```python
from build123d import *

# Parameters (mm, degrees)
F0_R     = 1.75
F0_R_2   = 2.75
F0_R_3   = 19.25
F1_DEPTH = 8
F2_R     = 3
F3_DEPTH = 3.5


with BuildPart() as f1:
    # F0 (on Right) → F1 (new body)
    with BuildSketch(Plane.YZ):
        with BuildLine():
            ThreePointArc((4.242641, 45.254834), (0, 47.012193), (-4.242641, 45.254834))
            Line((-4.242641, 45.254834), (-45.254834, 4.242641))
            ThreePointArc((-45.254834, 4.242641), (-47.012193, 0), (-45.254834, -4.242641))
            Line((-45.254834, -4.242641), (-4.242641, -45.254834))
            ThreePointArc((-4.242641, -45.254834), (0, -47.012193), (4.242641, -45.254834))
            Line((4.242641, -45.254834), (45.254834, -4.242641))
            ThreePointArc((45.254834, -4.242641), (47.012193, 0), (45.254834, 4.242641))
            Line((45.254834, 4.242641), (4.242641, 45.254834))
        make_face()
        with Locations((-24.5, -17.25)):
            Circle(F0_R, mode=Mode.SUBTRACT)
        with Locations((0, -33.3)):
            Circle(F0_R_2, mode=Mode.SUBTRACT)
        with Locations((24.5, -17.25)):
            Circle(F0_R, mode=Mode.SUBTRACT)
        with Locations((-33.3, 0)):
            Circle(F0_R_2, mode=Mode.SUBTRACT)
        with Locations((-24.5, 17.25)):
            Circle(F0_R, mode=Mode.SUBTRACT)
        Circle(F0_R_3, mode=Mode.SUBTRACT)
        with Locations((33.3, 0)):
            Circle(F0_R_2, mode=Mode.SUBTRACT)
        with Locations((24.5, 17.25)):
            Circle(F0_R, mode=Mode.SUBTRACT)
        with Locations((0, 33.3)):
            Circle(F0_R_2, mode=Mode.SUBTRACT)
    extrude(amount=F1_DEPTH)

    # F2 (on face) → F3 (cut)
    with BuildSketch(Plane(origin=(0, 0, 0), x_dir=(0, -1, 0), z_dir=(-1, 0, 0))):
        with Locations((24.5, 17.25)):
            Circle(F2_R)
        with Locations((-24.5, 17.25)):
            Circle(F2_R)
        with Locations((-24.5, -17.25)):
            Circle(F2_R)
        with Locations((24.5, -17.25)):
            Circle(F2_R)
    extrude(amount=-F3_DEPTH, mode=Mode.SUBTRACT)


solid = f1.part
```
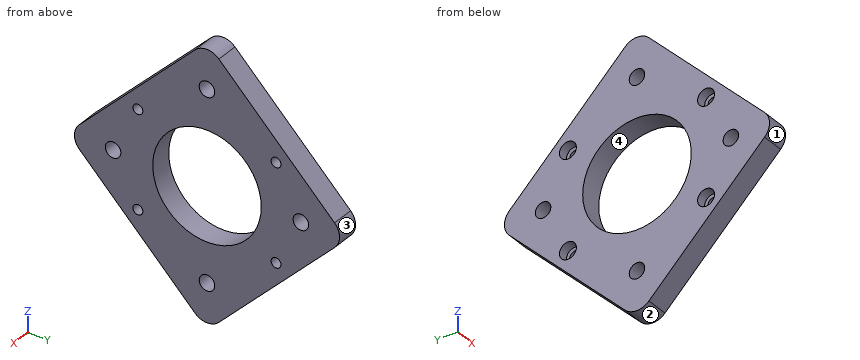
Design review of the part built by this model. Coordinates are the model's own, in mm. Face numbers are marked on the shaded views. Coordinates: 2 decimals unless noted, no trailing zeros. Write each loop counter-clockwise with the first axis right and the second up, starting at its lowest first coordinate (ties: lowest second). Pieces come first, ordered by that corner, then holes.
1) Add section B-B (y = -33.3). Write out the cut boundary in (x, z).
2) Add section A-A (z = 0). Write out the cut boundary in (x, y), plus the area to 3 significant figures.
3) To check wall thickness, follow L1, parallel to Y at x = 5.1, z = -17.25; L2, parallel to Y at x = 3.25, z = 0.5; L3, parallel to Z at x = 5.5, y = -24.5. State the ranges of each line that lie inside material, in increasing order.
4) Mouldability with a two-part tool opening along Y and no side actions: class the marked faces 1, 2, 3 and 4 as +Y half, -Y half, draft (parallel to the pull), parting line (faces both ways), or undercut.
5) Add section D-D (y = 29). Write out the cut boundary in (x, z), plus the area to 3 significant figures.
6) Insertion check: pin 1 (1.5 mm diameter, centred on x = 2, z = 28, fed in from -Y); pin 2 (4.5 mm diameter, centred on y = 24.5, z = -17.25, fed in from -X); pin 3 (1.5 mm diameter, centred on x = 2, y = 28.5, fed in from -Z); pin 4 (2 mm diameter, centred on y = -24.5, z = 17.25, fed in from -X). Each pin has a flat end and moves straight along its axis. Give the tip position at first contact, or say it passes through.
Check result:
1. outline: (0, -16.2) - (8, -16.2) - (8, -2.75) - (0, -2.75) - close; (0, 2.75) - (8, 2.75) - (8, 16.2) - (0, 16.2) - close
2. outline: (0, -47.01) - (8, -47.01) - (8, -36.05) - (0, -36.05) - close; (0, -30.55) - (8, -30.55) - (8, -19.25) - (0, -19.25) - close; (0, 19.25) - (8, 19.25) - (8, 30.55) - (0, 30.55) - close; (0, 36.05) - (8, 36.05) - (8, 47.01) - (0, 47.01) - close
2. area: 356 mm2
3. L1: y = -32.25 to -26.25, -22.75 to -8.54, 8.54 to 22.75, 26.25 to 32.25
3. L2: y = -46.99 to -36, -30.6 to -19.24, 19.24 to 30.6, 36 to 46.99
3. L3: z = -25 to -19, -15.5 to 15.5, 19 to 25
4. face 1: -Y half
4. face 2: parting line
4. face 3: +Y half
4. face 4: undercut
5. outline: (0, -20.5) - (8, -20.5) - (8, 20.5) - (0, 20.5) - close
5. area: 328 mm2
6. pin 1: stops at y = -22.25
6. pin 2: stops at x = 3.5
6. pin 3: stops at z = -21.75
6. pin 4: passes through
